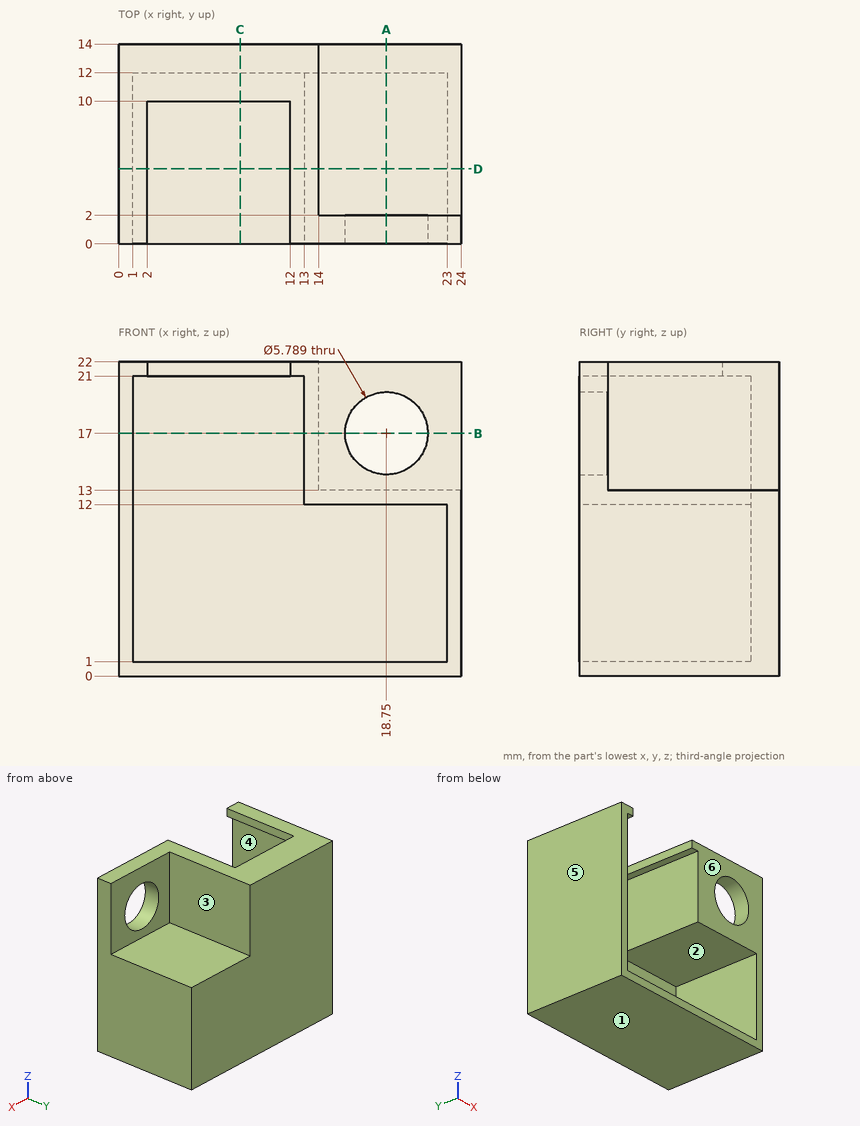
Geometry: see drawing. Coordinates: mm, zero at the bounding-box minimum. A direction names the side the tool comes from. Give positions to 0.01 mm unless a question says otherwise; leave off trailing zeros. Write each loop counter-clockwise with the first axis right and the second up, starting at its lowest first coordinate (ties: lowest second). Pieces come first, ordered by that corner, then holes. Notation, with made-up numbers: (-4.5, 36.25) -> (26.5, 36.25) arc R36 cw to (26.5, 73.25) -> close; hole circle Ø1 at (59, 47.5). An arc over 180 degrees is marked (long way). Use one line per item in the form item = value. Start each with the question number.
1) Pin query (flat end, axial travel): pin 1 (4.5 mm diameter, centred on y = 9.5, z = 17.5, fed in from +X); pin 2 (5 mm diameter, centred on x = 17, y = 5, fed in from +Z); pin 3 (3.5 mm diameter, centred on x = 7.5, y = 3.5, fed in from +Z). Return the tip coordinate at first contact, or that it passes through.
2) Section query C-C on x = 8.5. Return the cut outline in (y, z), then the cut area to 3 significant figures.
3) Section query D-D on y = 5.25. Return the cut outline in (x, z).
4) Set-up query: the marked faces 1, 2 and 3. Return all of +Z, -Z, +X, -X, +Y, -Y with unobstructed straight access to the full face (end or side cutting, diameter ignored); none if empty.
5) Section query A-A on x = 18.75. Return the cut outline in (y, z) (1 decimal).
6) Section query B-B on z = 17. Return the cut outline in (x, y) (1 decimal).
7) Ray query, probe 1 along Z at (x, y) = (18.75, 1.25) (1 decimal); probe 2 along X at (y, z) = (0.7, 17) (1 decimal); probe 3 along X at (y, z) = (6.25, 4). Return the intervals inside material, ascending. Write a range as from..to.
8) Draft query along X for the marked faces 4, 5 and 6. Return one class per face: pulls with the +X half, pulls with the -X half, needs draft (parallel to the pull), parting line crosses it, or undercut.
Outcome:
q1.pin_1 = 14
q1.pin_2 = 13
q1.pin_3 = 1
q2.outline = (0, 0) -> (14, 0) -> (14, 22) -> (10, 22) -> (10, 21) -> (12, 21) -> (12, 1) -> (0, 1) -> close
q2.area = 58.0 mm^2
q3.outline = (0, 0) -> (24, 0) -> (24, 13) -> (14, 13) -> (14, 22) -> (12, 22) -> (12, 21) -> (13, 21) -> (13, 12) -> (23, 12) -> (23, 1) -> (1, 1) -> (1, 21) -> (2, 21) -> (2, 22) -> (0, 22) -> close
q4.face_1 = -Z, +X, -X, +Y, -Y
q4.face_2 = -Y
q4.face_3 = +Z, +X, +Y
q5.outline = (0, 0) -> (14, 0) -> (14, 13) -> (2, 13) -> (2, 14.1) -> (0, 14.1) -> (0, 12) -> (12, 12) -> (12, 1) -> (0, 1) -> close; (0, 19.9) -> (2, 19.9) -> (2, 22) -> (0, 22) -> close
q6.outline = (0, 0) -> (1, 0) -> (1, 12) -> (13, 12) -> (13, 0) -> (15.9, 0) -> (15.9, 2) -> (14, 2) -> (14, 14) -> (0, 14) -> close; (21.6, 0) -> (24, 0) -> (24, 2) -> (21.6, 2) -> close
q7.probe_1 = 0..1, 12..14.1, 19.9..22
q7.probe_2 = 0..1, 13..15.9, 21.6..24
q7.probe_3 = 0..1, 23..24
q8.face_4 = undercut
q8.face_5 = pulls with the -X half
q8.face_6 = needs draft
